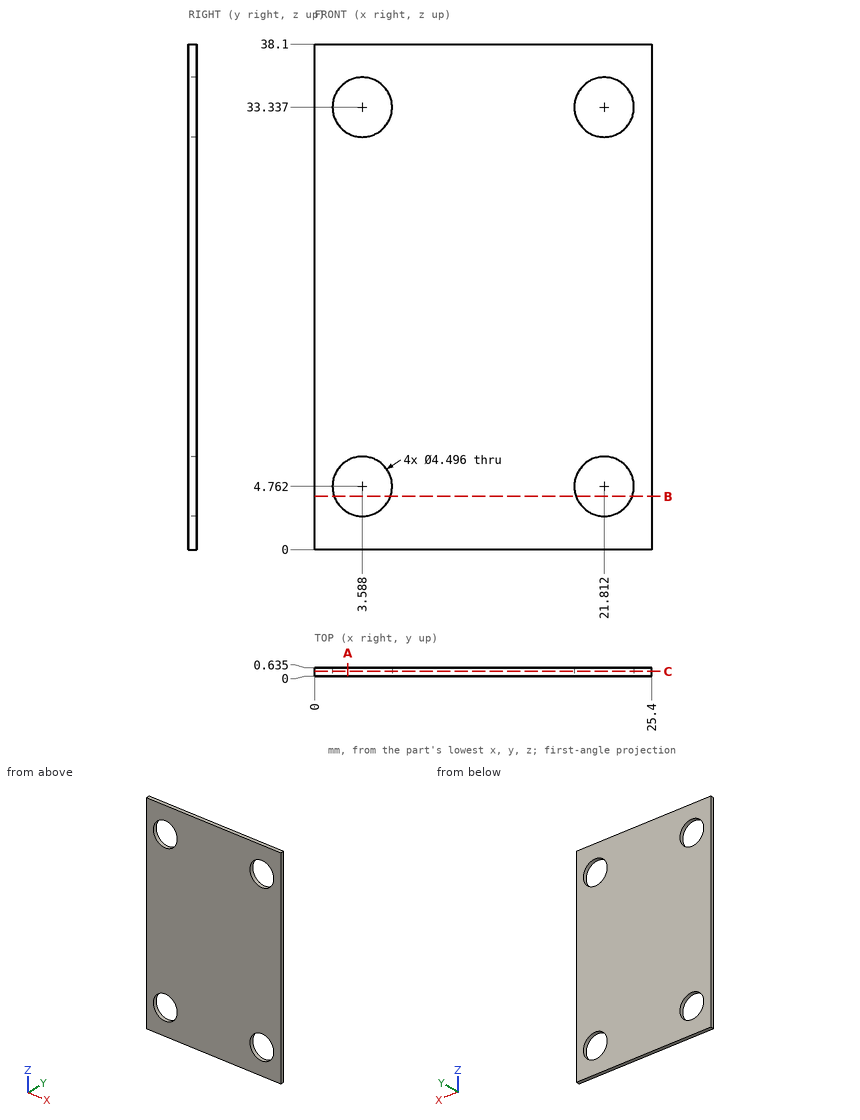
The drawing under review shows one solid part. Ordinate dimensions are in mm from its lowest x, y, z. Round coordinates to 2 decimals unless told otherwise and drop trailing zeros. Loops run counter-clockwise (first coordinate to the right, second up) from the corner with the lowest first, then second, coordinate; pieces in that order, holes last. Notation, with made-up numbers: (63, -13.75) - (72, -13.75) arc R31 cw to (72, 23.25) - close; hole circle Ø6 at (8.25, 49). An arc over 180 degrees is marked (long way). Use a Markdown table: item, result. Add a question column.
Q1. Add section A-A (x = 2.5). State the section outline as (y, z) points (1 decimal).
Q2. Insertion check: pin 1 Ø4 at (x, z) = (21.81, 4.76) entering from +Y. The pin has a flat end and moves straight along its axis. Give the tip position at first contact, or say it passes through.
Q3. Add section C-C (y = 0.35). State the section outline as (x, z) points (1 decimal), plus the area to 3 significant figures.
Q4. For probe 1 along Z at (x, y) = (21.75, 0.2) (1 decimal); probe 2 along X at (y, z) = (0.25, 3) (1 decimal); probe 3 along X at (y, z) = (0.2, 33) (1 decimal), list the stretches that pass through material, from the lowest coordinate up.
Q5. Add section B-B (z = 4). State the section outline as (x, y) points (1 decimal).
Worked answers:
| question | item | result |
|---|---|---|
| 1 | outline | (0, 0) - (0.6, 0) - (0.6, 2.8) - (0, 2.8) - close; (0, 6.7) - (0.6, 6.7) - (0.6, 31.4) - (0, 31.4) - close; (0, 35.3) - (0.6, 35.3) - (0.6, 38.1) - (0, 38.1) - close |
| 2 | pin 1 | through |
| 3 | outline | (0, 0) - (25.4, 0) - (25.4, 38.1) - (0, 38.1) - close; hole circle Ø4.5 at (3.6, 4.8); hole circle Ø4.5 at (3.6, 33.3); hole circle Ø4.5 at (21.8, 4.8); hole circle Ø4.5 at (21.8, 33.3) |
| 3 | area | 904 mm² |
| 4 | probe 1 | 0 to 2.5, 7 to 31.1, 35.6 to 38.1 |
| 4 | probe 2 | 0 to 2.2, 5 to 20.4, 23.2 to 25.4 |
| 4 | probe 3 | 0 to 1.4, 5.8 to 19.6, 24 to 25.4 |
| 5 | outline | (0, 0) - (1.5, 0) - (1.5, 0.6) - (0, 0.6) - close; (5.7, 0) - (19.7, 0) - (19.7, 0.6) - (5.7, 0.6) - close; (23.9, 0) - (25.4, 0) - (25.4, 0.6) - (23.9, 0.6) - close |
